Geometry check sheet. Reference: the model listing, model coordinates, mm. A direction names the side the tool comes from. Coordinates: 2 decimals unless noted, no trailing zeros. Write each loop counter-clockwise with the first axis right and the second up, starting at its lowest first coordinate (ties: lowest second). Pieces come first, ordered by that corner, then holes. Notation, with made-up numbers: (-21, 84) -> (21, 84) arc R25 ccw to (21, 106) -> close; hole circle Ø6 at (88, -14). An arc over 180 degrees is marked (long way). Answer as CSV lines item,"result".
```python
from build123d import *

# Parameters (mm, degrees)
SKETCH1_W           = 17
SKETCH1_H           = 67
BOSS_EXTRUDE1_DEPTH = 4
SKETCH2_W           = 12.5
SKETCH2_H           = 63.38
BOSS_EXTRUDE2_DEPTH = 5
SKETCH3_R           = 3.45
CUT_EXTRUDE1_DEPTH  = 1
SKETCH4_R           = 2.95
CUT_EXTRUDE2_DEPTH  = 7.5


with BuildPart() as part:
    # Sketch1 → Boss-Extrude1 (new body)
    with BuildSketch(Plane(origin=(0, 0, 0), x_dir=(1, 0, 0), z_dir=(0, 1, 0))):
        Rectangle(SKETCH1_W, SKETCH1_H)
    extrude(amount=BOSS_EXTRUDE1_DEPTH)

    # Sketch2 → Boss-Extrude2 (add)
    with BuildSketch(Plane(origin=(0, 4, 0), x_dir=(1, 0, 0), z_dir=(0, 1, 0))):
        Rectangle(SKETCH2_W, SKETCH2_H)
    extrude(amount=BOSS_EXTRUDE2_DEPTH)

    # Sketch3 → Cut-Extrude1 (cut)
    with BuildSketch(Plane.XZ):
        with Locations(Location((0, 0, 0), (0, 0, 270))):
            Circle(SKETCH3_R)
        with Locations(Location((0.136814879, 12.999280045, 0), (0, 0, 270))):
            Circle(SKETCH3_R)
        with Locations(Location((0.273629759, 25.99856009, 0), (0, 0, 270))):
            Circle(SKETCH3_R)
        with Locations(Location((0.000272251, -12.999999997, 0), (0, 0, 270))):
            Circle(SKETCH3_R)
        with Locations(Location((0.000544502, -25.999999994, 0), (0, 0, 270))):
            Circle(SKETCH3_R)
    extrude(amount=-CUT_EXTRUDE1_DEPTH, mode=Mode.SUBTRACT)

    # Sketch4 → Cut-Extrude2 (cut)
    with BuildSketch(Plane.XZ):
        with Locations(Location((0, 0, 0), (0, 0, 270))):
            Circle(SKETCH4_R)
        with Locations(Location((0.136814879, 12.999280045, 0), (0, 0, 270))):
            Circle(SKETCH4_R)
        with Locations(Location((0.273629759, 25.99856009, 0), (0, 0, 270))):
            Circle(SKETCH4_R)
        with Locations(Location((0.000272251, -12.999999997, 0), (0, 0, 270))):
            Circle(SKETCH4_R)
        with Locations(Location((0.000544502, -25.999999994, 0), (0, 0, 270))):
            Circle(SKETCH4_R)
    extrude(amount=-CUT_EXTRUDE2_DEPTH, mode=Mode.SUBTRACT)


solid = part.part
```
Item 1: Cross-section at D-D, the plane z = -13. Record the cut outline in (x, y).
Responses:
outline,"(-8.5, 0) -> (-3.45, 0) -> (-3.45, 1) -> (-2.95, 1) -> (-2.95, 7.5) -> (2.95, 7.5) -> (2.95, 1) -> (3.45, 1) -> (3.45, 0) -> (8.5, 0) -> (8.5, 4) -> (6.25, 4) -> (6.25, 9) -> (-6.25, 9) -> (-6.25, 4) -> (-8.5, 4) -> close"
Item 2: Cross-section at B-B, the plane y = 2.75. Record the cut outline in (x, z).
Responses:
outline,"(-8.5, -33.5) -> (8.5, -33.5) -> (8.5, 33.5) -> (-8.5, 33.5) -> close; hole circle Ø5.9 at (0, -26); hole circle Ø5.9 at (0, -13); hole circle Ø5.9 at (0, 0); hole circle Ø5.9 at (0.14, 13); hole circle Ø5.9 at (0.27, 26)"
Item 3: Thickness scan on probe 1 along X at (y, z) = (0.6, -13); probe 2 along Z at (x, y) = (0.75, 3.5); probe 3 along X at (y, z) = (7.25, 26.5). Record the ranges inside material, lowest first.
Responses:
probe 1,"x = -8.5 to -3.45, 3.45 to 8.5"
probe 2,"z = -33.5 to -28.85, -23.15 to -15.85, -10.15 to -2.85, 2.85 to 10.11, 15.88 to 23.09, 28.91 to 33.5"
probe 3,"x = -6.25 to -2.63, 3.18 to 6.25"
Item 4: Cross-section at A-A, the plane z = 5. Record the cut outline in (x, y).
Responses:
outline,"(-8.5, 0) -> (8.5, 0) -> (8.5, 4) -> (6.25, 4) -> (6.25, 9) -> (-6.25, 9) -> (-6.25, 4) -> (-8.5, 4) -> close"
Item 5: Set-up check for faces 5 (the flat face through (-6.25, 6, 0)), 6 (the flat face through (0, 9, 0)), 7 (the cylindrical face through (2.1, 4.2, 15.2)), 8 (the flat face through (0, 6, -31.69)): record each of +Z, -Z, +X, -X, +Y, -Y from which the full face is reachable in a straight line by a thin tool's end or side.
Responses:
face 5,"+Z, -Z, -X, +Y"
face 6,"+Z, -Z, +X, -X, +Y"
face 7,"-Y"
face 8,"-Z, +X, -X, +Y"
Item 6: Release check for a two-part mould opening along X. For faces 1 (the flat face through (4, 0, 0)), 2 (the flat face through (-8.5, 2, 0)), 3 (the flat face through (1, 1, -29)), 4 (the cylindrical face through (0.13, 4.204, -23.053)) record: +X half, -X half, draft (parallel to the pull), parting line (faces both ways), or undercut.
Responses:
face 1,"draft"
face 2,"-X half"
face 3,"undercut"
face 4,"undercut"
Item 7: Cross-section at C-C, the plane x = -4.25. Record the cut outline in (y, z), plus the area to 3 significant figures.
Responses:
outline,"(0, -33.5) -> (4, -33.5) -> (4, -31.69) -> (9, -31.69) -> (9, 31.69) -> (4, 31.69) -> (4, 33.5) -> (0, 33.5) -> close"
area,"585 mm2"
Item 8: Depth check by flat-ended pin: pin 1 Ø2.5 at (x, y) = (-0.5, 5.5) entering from +Z; pin 2 Ø2 at (x, z) = (-0.5, -27) entering from -Y; pin 3 Ø3 at (y, z) = (6, -8) entering from -X. Enter the tip coordinate at first touch or a pass-through.
Responses:
pin 1,"stops at z = 31.69"
pin 2,"stops at y = 7.5"
pin 3,"stops at x = -6.25"
